Here's how the part is built. I have some questions about the finished solid (model axes, mm). A direction names the side the tool comes from. Round coordinates to 2 decimals unless told otherwise and drop trailing zeros. Write each loop counter-clockwise with the first axis right and the second up, starting at its lowest first coordinate (ties: lowest second). Pieces come first, ordered by that corner, then holes. Notation, with made-up numbers: (48, 40.5) - (54, 40.5) arc R11 ccw to (54, 55.5) - close; hole circle Ø11 at (-40, -38.75). An arc over 180 degrees is marked (long way). Use one line per item in the form item = value. Start each with the question number.
1. I want a section at B-B, the plane z = 28. List the corners of the cut face in (x, y) for me.
2. I want a section at A-A, the plane y = 23. List the corners of the cut face in (x, z) for me (1 decimal), plus the area to 3 significant figures.
3. I want a section at C-C, the plane x = -47. List the corners of the cut face in (y, z) for me, plus the area to 3 significant figures.
4. Will these pins go through, and if not, where does the flat tip stop? pin 1 (20.5 mm diameter, centred on x = -54, y = 20.26, fed in from -Z); pin 2 (4 mm diameter, centred on x = -16, z = -2, fed in from -Y); pin 3 (10 mm diameter, centred on y = 46, z = 40, fed in from -X); pin 4 (6 mm diameter, centred on x = -30, z = -36, fed in from +Y).
5. If I drill on line 1 along X through (y, z) = (22, 49); line 2 along X through (y, z) = (-8, 49.5); line 3 along X through (y, z) = (21.5, -14.5), over which ranges is the centre line in solid material (lowest first)?
6. I want a section at D-D, the plane y = 4. List the corners of the cut face in (x, z) for me, plus the area to 3 significant figures.
7. Which directions (+Z, -Z, +X, -X, +Y, -Y) give clear straight access to the entire face, cutting with the end or side of a thin tool? Please do faces 1 (the flat face through (-43.7, 26.4, 55.097)), 2 (the flat face through (-1, 39, 4)).
8. We'd pull the mould along Y, two halves only. Please class faces 3 (the flat face through (-1, 0, 4)), 4 (the cylindrical face through (-47.87, 29.88, 3.84)), 5 (the flat face through (33, 26, 55.097)), 6 (the flat face through (3, 73, 30)): +Y half, -Y half, draft (parallel to the pull), parting line (faces both ways), or undercut.
```python
from build123d import *

# Parameters (mm, degrees)
F1_DEPTH = 19
F2_DEPTH = 92
F3_DEPTH = 39
F4_R     = 11.4088376228
F6_DEPTH = 103.9623373578
F5_R     = 12.6645604818
F7_DEPTH = 103.9623373578


with BuildPart() as f1:
    # F0 (on Front) → F1 (new body)
    with BuildSketch(Plane.XZ):
        with BuildLine():
            Line((-24.5031490922, 55.0966747105), (-31.5849818289, 55.0966747105))
            ThreePointArc((-31.5849818289, 55.0966747105), (-3.3992808312, 20.4304908119), (24.7864201665, 55.0966747105))
            Line((24.7864201665, 55.0966747105), (15.7216750085, 55.0966747105))
            ThreePointArc((15.7216750085, 55.0966747105), (-4.3907370418, 29.7217311132), (-24.5031490922, 55.0966747105))
        make_face()
    extrude(amount=F1_DEPTH)

    # F2 (add): a face of the model
    f2_faces = [f1.faces().sort_by_distance(p)[0] for p in [
        (20.2540475875, -19, 54.4245489648),
    ]]
    extrude(f2_faces, amount=-F2_DEPTH)

    # F0 (on Front) → F3 (join)
    with BuildSketch(Plane.XZ):
        with BuildLine():
            Line((-31.5849818289, 55.0966747105), (-74.6425390244, 55.0966747105))
            Line((-74.6425390244, 55.0966747105), (-74.6425390244, -48.8646626472))
            Line((-74.6425390244, -48.8646626472), (74.6425390244, -48.8646626472))
            Line((74.6425390244, -48.8646626472), (74.6425390244, 55.0966747105))
            Line((74.6425390244, 55.0966747105), (24.7864201665, 55.0966747105))
            ThreePointArc((24.7864201665, 55.0966747105), (-3.3992808312, 20.4304908119), (-31.5849818289, 55.0966747105))
        make_face()
    extrude(amount=-F3_DEPTH)

    # F4 (on face) → F6 (cut, through all)
    with BuildSketch(Plane.XY.offset(55.0966747105)):
        with Locations((-54.0047772229, 20.259199664)):
            Circle(F4_R)
    extrude(amount=-F6_DEPTH, mode=Mode.SUBTRACT)

    # F5 (on face) → F7 (cut, through all)
    with BuildSketch(Plane.XY.offset(55.0966747105)):
        with Locations((47.5070998073, 19.0783925354)):
            Circle(F5_R)
    extrude(amount=-F7_DEPTH, mode=Mode.SUBTRACT)


solid = f1.part
```
Model answer:
q1.outline = (-74.64, 0) - (-22.86, 0) - (-22.86, -19) - (16.06, -19) - (16.06, 0) - (74.64, 0) - (74.64, 39) - (16.06, 39) - (16.06, 73) - (-22.86, 73) - (-22.86, 39) - (-74.64, 39) - close; hole circle Ø22.82 at (-54, 20.26); hole circle Ø25.33 at (47.51, 19.08)
q2.outline = (-74.6, -48.9) - (-65.1, -48.9) - (-65.1, 55.1) - (-74.6, 55.1) - close; (-42.9, -48.9) - (35.5, -48.9) - (35.5, 55.1) - (15.7, 55.1) arc R20.7 cw (long way) to (-24.5, 55.1) - (-42.9, 55.1) - close; (59.5, -48.9) - (74.6, -48.9) - (74.6, 55.1) - (59.5, 55.1) - close
q2.area = 9,850 mm2
q3.outline = (0, -48.86) - (11.25, -48.86) - (11.25, 55.1) - (0, 55.1) - close; (29.26, -48.86) - (39, -48.86) - (39, 55.1) - (29.26, 55.1) - close
q3.area = 2,180 mm2
q4.pin_1 = through
q4.pin_2 = 0
q4.pin_3 = -31.88
q4.pin_4 = 39
q5.line_1 = -74.64 to -65.28, -42.73 to -25, 16.22 to 35.18, 59.83 to 74.64
q5.line_2 = -32.19 to -25.03, 16.25 to 25.39
q5.line_3 = -74.64 to -65.35, -42.66 to 35.08, 59.94 to 74.64
q6.outline = (-74.64, -48.86) - (74.64, -48.86) - (74.64, 55.1) - (15.72, 55.1) arc R20.66 cw (long way) to (-24.5, 55.1) - (-74.64, 55.1) - close
q6.area = 14,700 mm2
q7.face_1 = +Z, +X, -X, +Y, -Y
q7.face_2 = -Z, +Y
q8.face_3 = -Y half
q8.face_4 = undercut
q8.face_5 = draft
q8.face_6 = +Y half
